Source: CAD feature listing. Evaluate the final solid. Frame: model axes, mm. Face numbers are marked on the shaded views. Round coordinates to 2 decimals unless told otherwise and drop trailing zeros. Order: outer loops, then holes, each group sorted by start corner. A loop starts at its lowest first (then second) coordinate and runs counter-clockwise, first axis right, second up.
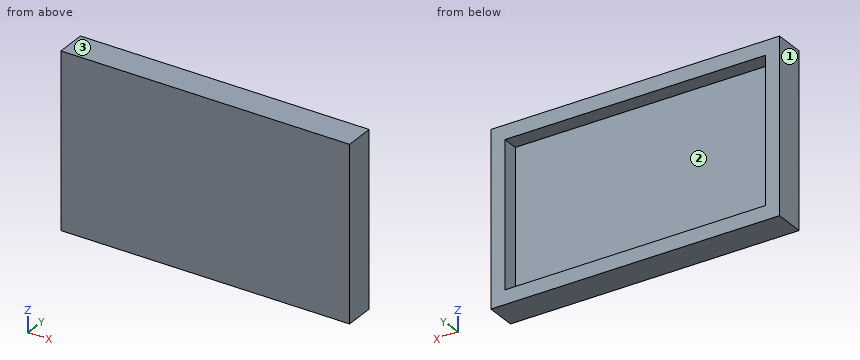
Autodesk Inventor part; units mm, degrees
ref_plane "YZ Plane" through (0, 0, 0) normal (1, 0, 0) x (0, 1, 0)
ref_plane "XZ Plane" through (0, 0, 0) normal (0, 1, 0) x (-1, 0, 0)
ref_plane "XY Plane" through (0, 0, 0) normal (0, 0, 1) x (1, 0, 0)
sketch "Sketch1" plane through (0, 0, 0) normal (0, 0, 1) x (1, 0, 0)
  line L0 (-9.8509, 0) -> (10.5499, 0)
  line L1 (10.5499, 0) -> (10.5499, -2.1187)
  line L2 (10.5499, -2.1187) -> (-9.8509, -2.1187)
  line L3 (-9.8509, -2.1187) -> (-9.8509, 0)
  point P0 (0, 0)
extrude "Extrusion1" add sketch "Sketch1" along normal blind 12.25
sketch "Sketch2" plane through (-9.8509, 0, 0) normal (0, 1, 0) x (1, 0, 0)
  line L0 (20.4008, 0) -> (0, 0)
  line L1 (0, 0) -> (0, -12.25)
  line L2 (20.4008, -12.25) -> (0, -12.25)
  line L3 (20.4008, 0) -> (20.4008, -12.25)
  line L4 (1.2669, -10.9831) -> (1.2669, -1.2669)
  line L5 (1.2669, -1.2669) -> (19.1339, -1.2669)
  line L6 (19.1339, -1.2669) -> (19.1339, -10.9831)
  line L7 (19.1339, -10.9831) -> (1.2669, -10.9831)
  point P0 (9.8509, 0)
  point P1 (9.3922, -1.2669)
  point P2 (9.3922, -10.9831)
shell "Shell1" thickness 1 removed faces 1 at (3.7496, 0, 4.0833)
properties part number "pan"
1. Line query: line 1 along X through (y, z) = (-0.35, 3.5); line 2 along Z through (x, y) = (-6, -0.9); line 3 along Y through (x, z) = (0.75, 6.75). Output: solid intervals per line, ascending.
2. Section C-C on x = 0.25. Return loops of the section in (y, z), plus the area to 3 significant figures.
3. First-contact query: pin 1 (2 mm diameter, centred on x = 5.5, z = 5.5, fed in from +Y). Flat tip, straight axial feed; report the tip coordinate or a pass-through.
4. Pull-direction query (Z, two-part tool) for the marked faces 1, 2 and 3; classes: released by +Z, released by -Z, zero draft, split by the parting line, or undercut.
5. Section A-A on z = 4.5. Return loops of the section in (x, y).
6. Section B-B on y = -0.75. Return loops of the section in (x, z), plus the area to 3 significant figures.
Result:
1. line 1: x = -9.85 to -8.85, 9.55 to 10.55
1. line 2: z = 0 to 1, 11.25 to 12.25
1. line 3: y = -2.12 to -1.12
2. outline: (-2.12, 0) - (0, 0) - (0, 1) - (-1.12, 1) - (-1.12, 11.25) - (0, 11.25) - (0, 12.25) - (-2.12, 12.25) - close
2. area: 14.5 mm2
3. pin 1: stops at y = -1.12
4. face 1: zero draft
4. face 2: undercut
4. face 3: released by +Z
5. outline: (-9.85, -2.12) - (10.55, -2.12) - (10.55, 0) - (9.55, 0) - (9.55, -1.12) - (-8.85, -1.12) - (-8.85, 0) - (-9.85, 0) - close
6. outline: (-9.85, 0) - (10.55, 0) - (10.55, 12.25) - (-9.85, 12.25) - close; hole (-8.85, 1) - (9.55, 1) - (9.55, 11.25) - (-8.85, 11.25) - close
6. area: 61.3 mm2
